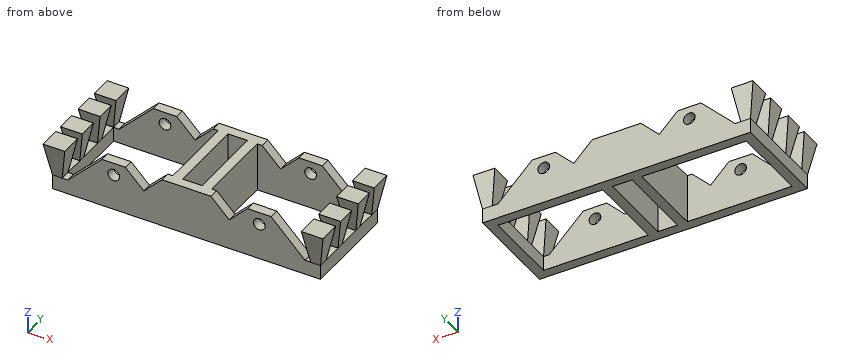
```python
from build123d import *

# Parameters (mm, degrees)
F0_R     = 1.25
F1_DEPTH = 20.8333333333
F2_W     = 22.3958333333
F2_H     = 16.6666666667
F2_W_2   = 4.1666666667
F3_DEPTH = 10.4176666667
F5_W     = 2.0833333333
F5_H     = 2.0833333333
F5_H_2   = 1.5
F6_DEPTH = 7.2916666667
F6_TAPER = -10


with BuildPart() as f1:
    # F0 (on Front) → F1 (new body)
    with BuildSketch(Plane.XZ):
        Polygon((-28.6458333333, 0), (0, 0), (28.6458333333, 0), (28.6458333333, 3.125), (25.3541666667, 3.125), (18.0625, 10.4166666667), (13.0625, 10.4166666667), (9.1354166667, 6.4895833333), (5.2083333333, 10.4166666667), (0, 10.4166666667), (-5.2083333333, 10.4166666667), (-9.1354166667, 6.4895833333), (-13.0625, 10.4166666667), (-18.0625, 10.4166666667), (-25.3541666667, 3.125), (-28.6458333333, 3.125), align=None)
        with Locations((-15.5625, 7.7708333333)):
            Circle(F0_R, mode=Mode.SUBTRACT)
        with Locations((15.5625, 7.7708333333)):
            Circle(F0_R, mode=Mode.SUBTRACT)
    extrude(amount=F1_DEPTH)

    # F2 (on face) → F3 (cut, through all)
    with BuildSketch(Plane.XY.offset(10.4166666667)):
        with Locations((-15.3645833333, -10.4166666667)):
            Rectangle(F2_W, F2_H)
        with Locations((15.3645833333, -10.4166666667)):
            Rectangle(F2_W, F2_H)
        with Locations((0, -10.4166666667)):
            Rectangle(F2_W_2, F2_H)
    extrude(amount=-F3_DEPTH, mode=Mode.SUBTRACT)

    # F5 (on offset) → F6 (join, through all)
    with BuildSketch(Plane.XY.offset(3.125)):
        with Locations((-27.6041666667, -1.0416666667)):
            Rectangle(F5_W, F5_H)
        with Locations((-27.6041666667, -19.7916666667)):
            Rectangle(F5_W, F5_H)
        with Locations((27.6041666667, -1.0416666667)):
            Rectangle(F5_W, F5_H)
        with Locations((27.6041666667, -19.7916666667)):
            Rectangle(F5_W, F5_H)
        with Locations((27.6041666667, -7.1666666667)):
            Rectangle(F5_W, F5_H_2)
        with Locations((27.6041666667, -13.6666666667)):
            Rectangle(F5_W, F5_H_2)
        with Locations((-27.6041666667, -7.1666666667)):
            Rectangle(F5_W, F5_H_2)
        with Locations((-27.6041666667, -13.6666666667)):
            Rectangle(F5_W, F5_H_2)
    extrude(amount=F6_DEPTH, taper=F6_TAPER)


solid = f1.part
```
Build history of the part. All positions in model axes, mm. Round coordinates to 2 decimals unless told otherwise and drop trailing zeros. Loops run counter-clockwise (first coordinate to the right, second up) from the corner with the lowest first, then second, coordinate; pieces in that order, holes last.
Item 1: Saw through at C-C (x = -10). List the corners of the cut face in (y, z).
Item 2: Pin check, flat tips, straight feed: P1, Ø2, axis at x = -15.56, z = 7.77, coming from the -Y side; P2, Ø4.5, axis at x = 1, z = 6.5, coming from the -Y side; P3, Ø6, axis at y = -15.5, z = 5.5, coming from the -X side; P4, Ø5, axis at y = -7, z = 6.5, coming from the +X side. Stop position of each tip, or through.
Item 3: Saw through at A-A (y = -4). List the corners of the cut face in (x, z) (1 decimal), then the cut area to 3 significant figures.
Item 4: Saw through at D-D (z = 9.75). State how many separate pieces and enclosed holes the cut face has, then the cut area to 3 significant figures.
Item 5: Saw through at B-B (z = 2.25). List the corners of the cut face in (x, y).
Item 6: Drill centre lines: line 1 along X through (y, z) = (-8.5, 2.75); line 2 along X through (y, z) = (-3, 6.5); line 3 along Y through (x, z) = (7, 7). Where is each one in solid material? Low to high.
Worked answers:
1. outline: (-20.83, 0) - (-18.75, 0) - (-18.75, 7.35) - (-20.83, 7.35) - close; (-2.08, 0) - (0, 0) - (0, 7.35) - (-2.08, 7.35) - close
2. P1: passes through
2. P2: stops at y = -20.83
2. P3: stops at x = -29.59
2. P4: stops at x = 29.68
3. outline: (-28.6, 0) - (-26.6, 0) - (-26.6, 3.1) - (-28.6, 3.1) - close; (-4.2, 0) - (-2.1, 0) - (-2.1, 10.4) - (-4.2, 10.4) - close; (2.1, 0) - (4.2, 0) - (4.2, 10.4) - (2.1, 10.4) - close; (26.6, 0) - (28.6, 0) - (28.6, 3.1) - (26.6, 3.1) - close
3. area: 56.4 mm2
4. separate pieces: 13
4. enclosed holes: 1
4. area: 317 mm2
5. outline: (-28.65, -20.83) - (28.65, -20.83) - (28.65, 0) - (-28.65, 0) - close; hole (-26.56, -18.75) - (-4.17, -18.75) - (-4.17, -2.08) - (-26.56, -2.08) - close; hole (-2.08, -18.75) - (2.08, -18.75) - (2.08, -2.08) - (-2.08, -2.08) - close; hole (4.17, -18.75) - (26.56, -18.75) - (26.56, -2.08) - (4.17, -2.08) - close
6. line 1: x = -28.65 to -26.56, -4.17 to -2.08, 2.08 to 4.17, 26.56 to 28.65
6. line 2: x = -4.17 to -2.08, 2.08 to 4.17
6. line 3: y = -20.83 to -18.75, -2.08 to 0
